The listing builds one solid part. Answer for the finished solid, in the listing's coordinates (mm). Face numbers are marked on the shaded views. A direction names the side the tool comes from. Give positions to 0.01 mm unless a question says otherwise; leave off trailing zeros. Write each loop counter-clockwise with the first axis right and the second up, starting at its lowest first coordinate (ties: lowest second). Pieces come first, ordered by that corner, then holes. Notation, with made-up numbers: (-7.5, 19.25) - (46.5, 19.25) arc R15 cw to (46.5, 32.25) - close; hole circle Ø7 at (29.25, -35). An arc over 180 degrees is marked (long way). Answer in a Markdown table with one row per item. Add a question column.
from build123d import *

# Parameters (mm, degrees)
BOSS_EXTRUDE1_DEPTH = 2
SKETCH2_R           = 2.75
BOSS_EXTRUDE2_DEPTH = 4
SKETCH2_3_R         = 2
CUT_EXTRUDE1_DEPTH  = 4
SKETCH3_R           = 3.5
BOSS_EXTRUDE3_DEPTH = 1
SKETCH3_4_R         = 2.5
BOSS_EXTRUDE4_DEPTH = 3
SKETCH4_R           = 2
CUT_EXTRUDE3_DEPTH  = 8.895146188
CHAMFER1_SIZE       = 0.2


with BuildPart() as part:
    # Sketch1 → Boss-Extrude1 (new body)
    with BuildSketch(Plane(origin=(0, 0, 0), x_dir=(1, 0, 0), z_dir=(0, 1, 0))):
        Polygon((0, 4.618802154), (-4, 2.309401077), (-4, -2.309401077), (0, -4.618802154), (4, -2.309401077), (4, 2.309401077), align=None)
    extrude(amount=BOSS_EXTRUDE1_DEPTH)

    # Sketch2 → Boss-Extrude2 (add)
    with BuildSketch(Plane(origin=(0, 2, 0), x_dir=(1, 0, 0), z_dir=(0, 1, 0))):
        with Locations(Location((0, 0, 0), (0, 0, 270))):
            Circle(SKETCH2_R)
    extrude(amount=BOSS_EXTRUDE2_DEPTH)

    # Sketch2_3 → Cut-Extrude1 (cut)
    with BuildSketch(Plane(origin=(0, 2, 0), x_dir=(1, 0, 0), z_dir=(0, 1, 0))):
        with Locations(Location((0, 0, 0), (0, 0, 270))):
            Circle(SKETCH2_3_R)
    extrude(amount=CUT_EXTRUDE1_DEPTH, mode=Mode.SUBTRACT)

    # Sketch3 → Boss-Extrude3 (add)
    with BuildSketch(Plane.XZ):
        with Locations(Location((0, 0, 0), (0, 0, 270))):
            Circle(SKETCH3_R)
    extrude(amount=BOSS_EXTRUDE3_DEPTH)

    # Sketch3_4 → Boss-Extrude4 (add)
    with BuildSketch(Plane.XZ):
        with Locations(Location((0, 0, 0), (0, 0, 270))):
            Circle(SKETCH3_4_R)
    extrude(amount=BOSS_EXTRUDE4_DEPTH)

    # Sketch4 → Cut-Extrude3 (cut, through all)
    with BuildSketch(Plane(origin=(0, 2, 0), x_dir=(1, 0, 0), z_dir=(0, 1, 0))):
        with Locations(Location((0, 0, 0), (0, 0, 270))):
            Circle(SKETCH4_R)
    extrude(amount=-CUT_EXTRUDE3_DEPTH, mode=Mode.SUBTRACT)

    # Chamfer1
    chamfer1_edges = [part.edges().sort_by_distance(p)[0] for p in [
        (0, 6, -2.75),
        (0, 6, -2),
        (0, -3, 2.5),
        (0, -3, -2),
    ]]
    chamfer(chamfer1_edges, length=CHAMFER1_SIZE)


solid = part.part
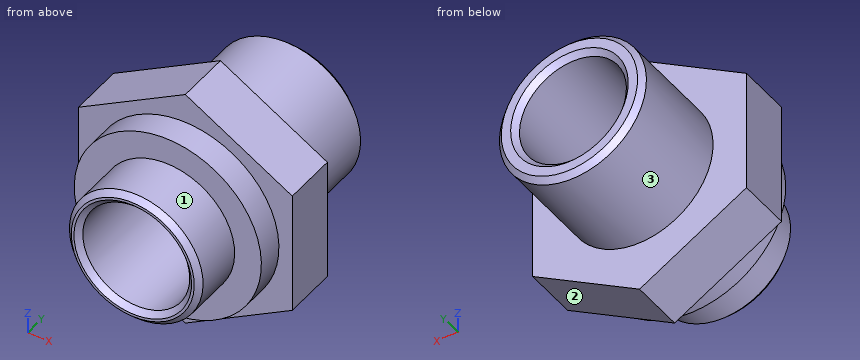
1. Given pin 1 Ø1 at (x, z) = (-1.5, -0.5) entering from +Y; pin 2 Ø2 at (x, z) = (1, 0.5) entering from -Y; pin 3 Ø1 at (x, y) = (1.5, 3) entering from -Z, each flat-ended and moving along its own axis, determine where each tip first touches the part or whether it passes through.
2. Section C-C (x = 3) is taken. Give the vertices of the cut face in (y, z).
3. A tool of negligible diameter and unlimited length cuts with its end or side. For the marked faces 1, 2 and 3, from which of +Z, -Z, +X, -X, +Y, -Y can it reach the whole face along a straight path? Write none if from no direction.
4. Section D-D (y = 3) is taken. Give the vertices of the cut face in (x, z), and give its area (3 significant figures).
5. Straight lines are drawn through the part: L1, parallel to X at y = -0.6, z = 0; L2, parallel to X at y = 4.15, z = 0; L3, parallel to Y at x = -2.25, z = 1.75. For each, find the intervals that lie inside material, in ascending order. Write a range as [from, to].
6. Section A-A (y = 0.75) is taken. Give the vertices of the cut face in (x, z).
7. Section B-B (z = 0) is taken. Give the vertices of the cut face in (x, y).
Geometry check:
| question | item | result |
|---|---|---|
| 1 | pin 1 | y = 5.88 |
| 1 | pin 2 | y = -2.92 |
| 1 | pin 3 | z = -2.56 |
| 2 | outline | (-1, -1.8) - (0, -1.8) - (0, -2.89) - (2, -2.89) - (2, 2.89) - (0, 2.89) - (0, 1.8) - (-1, 1.8) - close |
| 3 | face 1 | -Y |
| 3 | face 2 | -Z, +X, +Y, -Y |
| 3 | face 3 | +Y |
| 4 | outline | circle Ø5.5 at (0, 0); hole circle Ø4 at (0, 0) |
| 4 | area | 11.2 mm² |
| 5 | L1 | [-3.5, -2], [2, 3.5] |
| 5 | L2 | [-2.75, -2], [2, 2.75] |
| 5 | L3 | [-1, 2] |
| 6 | outline | (-4, -2.31) - (0, -4.62) - (4, -2.31) - (4, 2.31) - (0, 4.62) - (-4, 2.31) - close; hole circle Ø4 at (0, 0) |
| 7 | outline | (-4, 0) - (-3.5, 0) - (-3.5, -1) - (-2.5, -1) - (-2.5, -2.8) - (-2.3, -3) - (-2.2, -3) - (-2, -2.8) - (-2, 5.8) - (-2.2, 6) - (-2.55, 6) - (-2.75, 5.8) - (-2.75, 2) - (-4, 2) - close; (2, -2.8) - (2.2, -3) - (2.3, -3) - (2.5, -2.8) - (2.5, -1) - (3.5, -1) - (3.5, 0) - (4, 0) - (4, 2) - (2.75, 2) - (2.75, 5.8) - (2.55, 6) - (2.2, 6) - (2, 5.8) - close |
